Autodesk Inventor part; units mm, degrees
ref_plane "YZ Plane" through (0, 0, 0) normal (1, 0, 0) x (0, 1, 0)
ref_plane "XZ Plane" through (0, 0, 0) normal (0, 1, 0) x (-1, 0, 0)
ref_plane "XY Plane" through (0, 0, 0) normal (0, 0, 1) x (1, 0, 0)
sketch "Sketch1" plane through (0, 0, 0) normal (0, 0, 1) x (1, 0, 0)
  line L0 (0, 35) -> (0, -35) construction
  line L1 (-35, 0) -> (35, 0) construction
  circle A0 centre (0, 0) radius 25
  dimension "d0" = 50
extrude "Extrusion1" add sketch "Sketch1" along normal blind 10
sketch "Sketch2" plane through (0, 0, 10) normal (0, 0, 1) x (1, 0, 0)
  point P0 (0, 0)
  point P1 (0, 0)
hole "Hole1" at (0, 0, 10) direction (0, 0, -1) diameter 4.917 end through all
sketch "Sketch3" plane through (0, 0, 10) normal (0, 0, 1) x (1, 0, 0)
  circle A0 centre (0, 0) radius 19 construction
  line L0 (0, 35) -> (0, -35) construction
  point P0 (0, 19)
  point P1 (-16.4545, -9.5)
  point P2 (16.4545, -9.5)
  dimension "d10" = 38
  dimension "d11" = 120
  dimension "d12" = 120
hole "Hole2" at (0, 19, 10) at (-16.4545, -9.5, 10) at (16.4545, -9.5, 10) direction (0, 0, -1) diameter 4 end through all counterbore diameter 7 counterbore depth 4
chamfer "Chamfer1" distance 1 angle 45 1 edges at (-25, 0, 10)
properties part number "M-060-Adapter"
Source: CAD feature listing. Evaluate the final solid. Frame: model axes, mm. A direction names the side the tool comes from. Give positions to 0.01 mm unless a question says otherwise; leave off trailing zeros. Loops run counter-clockwise (first coordinate to the right, second up) from the corner with the lowest first, then second, coordinate; pieces in that order, holes last. Notation, with made-up numbers: M 43,42.5 L 62,42.5 A20 ccw 62,51.5 Z; hole C 58,-36 d6. An arc over 180 degrees is marked long. Put each result on its own line as item: value.
Q1. Section A-A (x = 0). Return the cut outline in (y, z), and give its area (3 significant figures).
Response values:
outline: M -25,0 L -2.46,0 L -2.46,10 L -24,10 L -25,9 Z; M 2.46,0 L 17,0 L 17,6 L 15.5,6 L 15.5,10 L 2.46,10 Z; M 21,0 L 25,0 L 25,9 L 24,10 L 22.5,10 L 22.5,6 L 21,6 Z
area: 398 mm²
Q2. Reachability of faces 4 (the cylindrical face through (1.2, 20.6, 3)), 5 (the cylindrical face through (16.301, -6.003, 7.972)) from +Z, -Z, +X, -X, +Y, -Y: full face, straight path, thin tool, end or side. Return the list, or none.
Response values:
face 4: +Z, -Z
face 5: +Z
Q3. Section B-B (z = 4.25). Return the cut outline in (x, y).
Response values:
outline: C 0,0 d50; hole C -16.45,-9.5 d4; hole C 0,0 d4.92; hole C 0,19 d4; hole C 16.45,-9.5 d4
Q4. Section C-C (y = -9.5). Count the separate pieces of the cut face and the enclosed holes in it, and give its area (3 significant figures).
Response values:
separate pieces: 3
enclosed holes: 0
area: 357 mm²
Q5. Mould query, pull axis X, two halves, no side actions, for faces 1 (the cylindrical face through (23.846, -7.509, 4.437)), 2 (the flat face through (0, -5, 10)), 3 (the cylindrical face through (-14.325, -6.723, 7.972)). Classes: released by +X, released by -X, zero draft, split by the parting line, or undercut.
Response values:
face 1: split by the parting line
face 2: zero draft
face 3: undercut
Q6. Line query: probe 1 along Y at (x, z) = (0, 5.25); probe 2 along Y at (x, z) = (0, 8.05); probe 3 along X at (y, z) = (-9.5, 4.6). Output: solid intervals per line, ascending. Write a range as [from, to].
Response values:
probe 1: y = [-25, -2.46], [2.46, 17], [21, 25]
probe 2: y = [-25, -2.46], [2.46, 15.5], [22.5, 25]
probe 3: x = [-23.12, -18.45], [-14.45, 14.45], [18.45, 23.12]
Q7. Pin query (flat end, axial travel): P1, Ø3.5, axis at x = -16, y = -8, coming from the +Z side; P2, Ø5, axis at x = 5.5, z = 7.5, coming from the +Y side; P3, Ø1, axis at y = 12.5, z = 3.5, coming from the -X side; P4, Ø3, axis at x = 0, y = 0, coming from the -Z side. Return the tip coordinate at first contact, or that it passes through.
Response values:
P1: stops at z = 6
P2: stops at y = 24.82
P3: stops at x = -21.93
P4: passes through
